Source: CAD feature listing. Evaluate the final solid. Frame: model axes, mm. A direction names the side the tool comes from. Give positions to 0.01 mm unless a question says otherwise; leave off trailing zeros. Order: outer loops, then holes, each group sorted by start corner. A loop starts at its lowest first (then second) coordinate and runs counter-clockwise, first axis right, second up.
Autodesk Inventor part; units mm, degrees
ref_plane "YZ Plane" through (0, 0, 0) normal (1, 0, 0) x (0, 1, 0)
ref_plane "XZ Plane" through (0, 0, 0) normal (0, 1, 0) x (-1, 0, 0)
ref_plane "XY Plane" through (0, 0, 0) normal (0, 0, 1) x (1, 0, 0)
sketch "Sketch1" plane through (0, 0, 0) normal (1, 0, 0) x (0, 1, 0)
  line L0 (444.5, 0) -> (444.5, -2.1042)
  line L1 (0, -2.1042) -> (0, 0)
  line L2 (0, -74.1174) -> (0, -66.8433)
  line L3 (0, 0) -> (82.55, 0)
  line L4 (82.55, 0) -> (82.55, -393.7)
  line L5 (82.55, -393.7) -> (0, -393.7)
  line L6 (0, -393.7) -> (0, 0)
  point P0 (25.4, -50.8)
  point P1 (25.4, -342.9)
  dimension "d2" = 82.55
  dimension "d3" = 393.7
  dimension "d4" = 50.8
  dimension "d5" = 25.4
  dimension "d6" = 50.8
  dimension "d7" = 25.4
extrude "Extrusion1" add sketch "Sketch1" along normal blind 6.35
sketch "Sketch3" plane through (6.35, 0, 0) normal (1, 0, 0) x (0, 0, -1)
  point P0 (0, 0)
sketch "Sketch4" plane through (6.35, 0, 0) normal (1, 0, 0) x (0, 0, -1)
  point P0 (0, 0)
chamfer "Chamfer1" distance 38.1 angle 45 1 edges at (3.175, 0, 0)
chamfer "Chamfer2" distance 38.1 angle 45 1 edges at (3.175, 0, -393.7)
sketch "Sketch5" plane through (0, 0, 0) normal (-1, 0, 0) x (0, 0, 1)
  line L0 (0, 82.55) -> (-393.7, 82.55)
  line L1 (-355.6, 0) -> (-393.7, 38.1)
  line L2 (-355.6, 0) -> (-38.1, 0)
  line L3 (0, 38.1) -> (-38.1, 0)
  line L4 (0, 38.1) -> (0, 82.55)
  line L5 (0, 82.55) -> (-393.7, 82.55)
  line L6 (-393.7, 82.55) -> (-393.7, 38.1)
  point P0 (0, 0)
  point P1 (-342.9, 38.1)
  point P2 (-50.8, 38.1)
  dimension "d16" = 50.8
  dimension "d17" = 38.1
  dimension "d18" = 38.1
  dimension "d19" = 50.8
hole "Hole1" at (0, 38.1, -342.9) at (0, 38.1, -50.8) direction (1, 0, 0) diameter 12.7254 end through all
sketch "Sketch7" plane through (0, 0, 0) normal (-1, 0, 0) x (0, 0, 1)
  line L0 (-38.1, 0) -> (-355.6, 0)
  line L1 (-393.7, 82.55) -> (-393.7, 38.1)
  line L2 (0, 38.1) -> (0, 82.55)
  line L3 (0, 82.55) -> (-393.7, 82.55)
  point P0 (0, 0)
  point P1 (-298.45, 10.0076)
  point P2 (-95.25, 10.0076)
  point P3 (-12.7, 78.8924)
  point P4 (-381, 78.8924)
  dimension "d42" = 10.0076
  dimension "d43" = 95.25
  dimension "d44" = 95.25
  dimension "d45" = 3.6576
  dimension "d46" = 12.7
  dimension "d47" = 12.7
  dimension "d82" = 3.6576
hole "Hole3" at (0, 78.8924, -381) at (0, 78.8924, -12.7) direction (1, 0, 0) diameter 4.7752 end through all
sketch "Sketch8" plane through (0, 0, 0) normal (-1, 0, 0) x (0, 0, 1)
  line L0 (0, 38.1) -> (0, 82.55)
  line L1 (0, 82.55) -> (-393.7, 82.55)
  line L2 (-355.6, 0) -> (-38.1, 0)
  line L3 (-393.7, 38.1) -> (-393.7, 82.55)
  point P0 (0, 0)
  point P1 (-171.45, 78.8924)
  point P2 (-222.25, 10.0076)
  dimension "d57" = 10.0076
  dimension "d128" = 222.25
hole "Hole4" at (0, 10.0076, -222.25) direction (1, 0, 0) diameter 3.556 end through all
sketch "Sketch10" plane through (0, 0, 0) normal (-1, 0, 0) x (0, 0, 1)
  circle A0 centre (-222.25, 44.45) radius 1.778
  circle A1 centre (-127, 44.45) radius 1.778
  line L0 (-393.7, 82.55) -> (0, 82.55)
  line L1 (-114.3619, 67.6125) -> (-112.4836, 67.6125)
  point P0 (0, 0)
  point P1 (-220.472, 44.45)
  point P2 (-128.778, 44.45)
  dimension "d108" = 38.1
  dimension "d109" = 38.1
hole "Hole6" at (0, 44.45, -127) at (0, 44.45, -220.472) at (0, 44.45, -128.778) at (0, 44.45, -222.25) direction (1, 0, 0) diameter 43.18 end through all
sketch "Sketch14" plane through (6.35, 0, 0) normal (1, 0, 0) x (0, 0, -1)
  arc A0 (127.889, 66.0217) -> (127.889, 22.8783) centre (127, 44.45) ccw
  arc A1 (127.889, 22.8783) -> (127.889, 66.0217) centre (128.778, 44.45) ccw
  arc A2 (221.361, 66.0217) -> (221.361, 22.8783) centre (220.472, 44.45) ccw
  arc A3 (221.361, 22.8783) -> (221.361, 66.0217) centre (222.25, 44.45) ccw
  line L0 (127.889, 66.0217) -> (127.889, 22.8783)
  line L1 (96.03, 44.45) -> (156.5626, 44.45)
  line L2 (221.361, 66.0217) -> (221.361, 22.8783)
  line L3 (190.5646, 36.322) -> (248.6345, 36.322)
  line L4 (127.889, 44.45) -> (103.886, 44.45)
  line L5 (103.886, 44.45) -> (103.886, 51.4604)
  line L6 (103.886, 51.4604) -> (103.886, 44.45)
  line L7 (103.886, 44.45) -> (103.886, 37.4396)
  line L8 (127.889, 44.45) -> (151.892, 44.45)
  line L9 (151.892, 44.45) -> (151.892, 37.4396)
  line L10 (151.892, 44.45) -> (151.892, 51.4604)
  line L11 (221.361, 51.4604) -> (197.358, 51.4604)
  line L12 (221.361, 51.4604) -> (245.364, 51.4604)
  line L13 (221.361, 37.4396) -> (197.358, 37.4396)
  line L14 (221.361, 37.4396) -> (245.364, 37.4396)
  circle A4 centre (103.886, 37.4396) radius 1.7526
  circle A5 centre (103.886, 51.4604) radius 1.7526
  circle A6 centre (151.892, 51.4604) radius 1.7526
  circle A7 centre (151.892, 37.4396) radius 1.7526
  circle A8 centre (197.358, 51.4604) radius 1.7526
  circle A9 centre (197.358, 37.4396) radius 1.7526
  circle A10 centre (245.364, 37.4396) radius 1.7526
  circle A11 centre (245.364, 51.4604) radius 1.7526
  point P0 (0, 0)
  dimension "d113" = 24.003
  dimension "d114" = 7.0104
  dimension "d115" = 7.0104
  dimension "d116" = 24.003
  dimension "d117" = 24.003
  dimension "d118" = 24.003
  dimension "d119" = 3.5052
  dimension "d120" = 3.5052
  dimension "d121" = 3.5052
  dimension "d122" = 3.5052
  dimension "d123" = 3.5052
extrude "Extrusion2" cut sketch "Sketch14" against normal blind 25.4 contours A9 L3 | A10 L3 | A9 L3 | L3 A10 | A4 | A5 | A6 | A7 | A8 | A11
thicken "Thicken1" operation add thickness 6.35 both sides no extend neighbours yes toward (0, 1, 0) faces at (2.1167, 82.55, -131.2333)
sketch "Sketch16" plane through (6.35, 0, 0) normal (1, 0, 0) x (0, 0, -1)
  line L0 (393.7, 88.9) -> (0, 88.9)
  line L1 (42.6019, 88.9) -> (52.7619, 88.9)
  line L2 (52.7619, 88.9) -> (52.7619, 78.74)
  line L3 (31.75, 78.74) -> (107.95, 78.74)
  line L4 (31.75, 78.74) -> (107.95, 78.74) construction
  point P0 (0, 0)
  dimension "d131" = 10.16
  dimension "d132" = 10.16
  dimension "d133" = 76.2
sketch "Sketch17" plane through (6.35, 0, 0) normal (1, 0, 0) x (0, 0, -1)
  circle A0 centre (139.7, 78.74) radius 1.778
  line L0 (393.7, 38.1) -> (393.7, 88.9)
  line L1 (393.7, 78.74) -> (304.8, 78.74)
  line L2 (393.7, 78.74) -> (482.6, 78.74) construction
  circle A1 centre (304.8, 78.74) radius 1.778
  point P0 (0, 0)
  dimension "d135" = 3.556
  dimension "d136" = 88.9
  dimension "d138" = 3.556
sketch "Sketch18" plane through (6.35, 0, 0) normal (1, 0, 0) x (0, 0, -1)
  line L0 (0, 0) -> (0, 10.0076)
  line L1 (0, 0) -> (10.0076, 0) construction
  line L2 (0, 10.0076) -> (101.6, 10.0076)
  line L3 (0, 10.0076) -> (101.6, 10.0076) construction
  line L4 (393.7, 10.0076) -> (292.1, 10.0076)
  line L5 (393.7, 10.0076) -> (495.3, 10.0076) construction
  circle A0 centre (101.6, 10.0076) radius 2.3876
  circle A1 centre (292.1, 10.0076) radius 2.3876
  dimension "d139" = 10.0076
  dimension "d141" = 101.6
  dimension "d143" = 101.6
  dimension "d145" = 4.7752
  dimension "d146" = 4.7752
hole "Hole10" at (6.35, 78.74, -107.95) direction (-1, 0, 0) diameter 3.556 depth 25.4 tip angle 118
hole "Hole11" at (6.35, 78.74, -304.8) direction (-1, 0, 0) diameter 3.556 depth 25.4 tip angle 118
hole "Hole12" at (6.35, 10.0076, -292.1) direction (-1, 0, 0) diameter 3.556 depth 25.4 tip angle 118
hole "Hole13" at (6.35, 10.0076, -101.6) direction (-1, 0, 0) diameter 3.556 depth 25.4 tip angle 118
sketch "Sketch19" plane through (6.35, 0, 0) normal (1, 0, 0) x (0, 0, -1)
  point P0 (0, 0)
sketch "Sketch20" plane through (6.35, 0, 0) normal (1, 0, 0) x (0, 0, -1)
  line L0 (0, 88.9) -> (0, 38.1)
  line L1 (38.1, 0) -> (0, 38.1)
  line L2 (38.1, 0) -> (355.6, 0)
  line L3 (393.7, 38.1) -> (355.6, 0)
  line L4 (393.7, 38.1) -> (393.7, 88.9)
  line L5 (393.7, 88.9) -> (0, 88.9)
  line L6 (0, 63.5) -> (19.05, 63.5)
  line L7 (19.05, 88.9) -> (19.05, 69.85)
  line L8 (56.4869, 0) -> (56.4869, 19.05)
  circle A0 centre (50.8, 38.1) radius 6.3627
  circle A1 centre (50.8, 38.1) radius 6.3627
  line L9 (44.4412, 37.8775) -> (33.0112, 37.8775)
  line L10 (50.5074, 44.456) -> (50.5074, 55.886)
  line L11 (57.1622, 38.1805) -> (68.5922, 38.1805)
  circle A2 centre (103.886, 37.4396) radius 1.7526
  line L12 (102.1334, 37.4396) -> (90.7034, 37.4396)
  line L13 (80.4606, 88.9) -> (80.4606, 69.85)
  line L14 (68.5922, 69.85) -> (90.7034, 69.85)
  line L15 (90.7034, 69.85) -> (90.7034, 19.05)
  line L16 (90.7034, 19.05) -> (68.5922, 19.05)
  line L17 (68.5922, 19.05) -> (68.5922, 69.85)
  line L18 (19.05, 69.85) -> (33.0112, 69.85)
  line L19 (33.0112, 69.85) -> (33.0112, 33.0112)
  line L20 (33.0112, 33.0112) -> (19.05, 33.0112)
  line L21 (19.05, 33.0112) -> (19.05, 69.85)
  line L22 (19.05, 33.0112) -> (33.0112, 33.0112)
  line L23 (33.0112, 33.0112) -> (33.0112, 19.05)
  line L24 (33.0112, 19.05) -> (19.05, 33.0112)
  line L25 (33.0112, 19.05) -> (33.0112, 33.0112)
  line L26 (19.05, 33.0112) -> (33.0112, 33.0112)
  line L27 (19.05, 33.0112) -> (33.0112, 19.05)
  line L28 (33.0112, 33.0112) -> (33.0112, 69.85)
  line L29 (33.0112, 69.85) -> (19.05, 69.85)
  line L30 (19.05, 69.85) -> (19.05, 33.0112)
  point P0 (0, 0)
  dimension "d183" = 19.05
  dimension "d184" = 19.05
  dimension "d185" = 19.05
  dimension "d186" = 11.43
  dimension "d187" = 11.43
  dimension "d188" = 11.43
  dimension "d189" = 11.43
  dimension "d190" = 19.05
extrude "Extrusion3" cut sketch "Sketch20" against normal blind 25.4 contours L14 L15 L16 L17
extrude "Extrusion4" cut sketch "Sketch20" against normal blind 25.4 contours L21 L18 L19 L20 | L20 L23 L24
sketch "Sketch21" plane through (6.35, 0, 0) normal (1, 0, 0) x (0, 0, -1)
  circle A0 centre (151.892, 51.4604) radius 1.7526
  line L0 (38.1, 0) -> (355.6, 0)
  circle A1 centre (197.358, 51.4604) radius 1.7526
  line L1 (393.7, 88.9) -> (0, 88.9)
  line L2 (0, 88.9) -> (393.7, 88.9)
  line L3 (175.7731, 88.9) -> (175.7731, 69.85)
  line L4 (153.6446, 51.4604) -> (165.0746, 51.4604)
  circle A2 centre (197.358, 51.4604) radius 1.7526
  line L5 (195.6055, 51.4771) -> (184.1755, 51.4771)
  line L6 (355.6, 0) -> (38.1, 0)
  line L7 (175.7731, 0) -> (175.7731, 19.05)
  line L8 (165.0746, 69.85) -> (184.1755, 69.85)
  line L9 (184.1755, 69.85) -> (184.1755, 19.05)
  line L10 (184.1755, 19.05) -> (165.0746, 19.05)
  line L11 (165.0746, 19.05) -> (165.0746, 69.85)
  circle A3 centre (245.364, 51.4604) radius 1.7526
  circle A4 centre (245.364, 37.4396) radius 1.7526
  circle A5 centre (342.9, 38.1) radius 6.3627
  line L12 (267.1323, 0) -> (267.1323, 19.05)
  line L13 (267.1323, 88.9) -> (267.1323, 69.85)
  line L14 (247.1166, 51.4604) -> (258.5466, 51.4604)
  line L15 (336.5373, 38.1) -> (325.1073, 38.1)
  line L16 (258.5466, 69.85) -> (325.1073, 69.85)
  line L17 (325.1073, 69.85) -> (325.1073, 19.05)
  line L18 (325.1073, 19.05) -> (258.5466, 19.05)
  line L19 (258.5466, 19.05) -> (258.5466, 69.85)
  point P0 (0, 0)
  dimension "d195" = 19.05
  dimension "d196" = 11.43
  dimension "d197" = 11.43
  dimension "d198" = 19.05
  dimension "d199" = 19.05
  dimension "d200" = 19.05
  dimension "d201" = 11.43
  dimension "d202" = 11.43
extrude "Extrusion5" cut sketch "Sketch21" against normal blind 25.4 contours L10 L11 L8 L9
extrude "Extrusion6" cut sketch "Sketch21" against normal blind 25.4 contours L18 L19 L16 L17
sketch "Sketch22" plane through (6.35, 0, 0) normal (1, 0, 0) x (0, 0, -1)
  line L0 (393.7, 38.1) -> (393.7, 88.9)
  line L1 (361.8045, 88.9) -> (361.8045, 69.85)
  circle A0 centre (342.9, 38.1) radius 6.3627
  line L2 (349.2627, 38.1) -> (360.6927, 38.1)
  line L3 (393.7, 39.2414) -> (374.65, 39.2414)
  line L4 (360.6927, 69.85) -> (374.65, 69.85)
  line L5 (374.65, 69.85) -> (374.65, 27.244)
  line L6 (374.65, 27.244) -> (360.6927, 27.244)
  line L7 (360.6927, 27.244) -> (360.6927, 69.85)
  line L8 (360.6927, 27.244) -> (360.6927, 13.2867)
  line L9 (360.6927, 13.2867) -> (374.65, 27.244)
  line L10 (355.6, 0) -> (393.7, 38.1)
  point P0 (0, 0)
  dimension "d207" = 19.05
  dimension "d208" = 11.43
  dimension "d209" = 19.05
extrude "Extrusion7" cut sketch "Sketch22" against normal blind 25.4 contours L4 L5 L6 L7 | L6 L9 L8
properties part number "DriveTrainPlate"
1) Ray query, L1, parallel to Z at x = 5.25, y = 68; L2, parallel to Z at x = 1.75, y = 9.5; L3, parallel to Y at x = 1.25, z = -79. Return the intervals inside material, ascending.
Checks:
L1: z = -393.7 to -374.65, -360.69 to -325.11, -258.55 to -184.18, -165.07 to -90.7, -68.59 to -33.01, -19.05 to 0
L2: z = -365.1 to -293.8, -290.4 to -223.95, -220.55 to -103.3, -99.9 to -28.6
L3: y = 0 to 19.05, 69.85 to 88.9
2) Section query A-A on z = -50.8. Output: boundary loops of the cut face in (x, y).
Checks:
outline: (0, 0) - (6.35, 0) - (6.35, 31.74) - (0, 31.74) - close; (0, 44.46) - (6.35, 44.46) - (6.35, 88.9) - (0, 88.9) - close
3) Section query B-B on z = -118. Output: boundary loops of the cut face in (x, y), and give its area (3 significant figures).
Checks:
outline: (0, 0) - (6.35, 0) - (6.35, 24.83) - (0, 24.83) - close; (0, 64.07) - (6.35, 64.07) - (6.35, 88.9) - (0, 88.9) - close
area: 315 mm2
4) Reachability of faces 4 (the face through (3, 69.85, -291)), 5 (the face through (0, 44, -194)) from +Z, -Z, +X, -X, +Y, -Y: full face, straight path, thin tool, end or side. Return the list, or none.
Checks:
face 4: +X, -X
face 5: +Z, -Z, -X, +Y, -Y
5) Pull-direction query (Z, two-part tool) for faces 1 (the face through (3.1, 18.8, -374.4)), 2 (the face through (3, 44, -258.547)), 3 (the face through (3, 0, -199)); classes: +Z half, -Z half, draft (parallel to the pull), parting line (faces both ways), or undercut.
Checks:
face 1: -Z half
face 2: undercut
face 3: draft
6) Section query C-C on x = 1.25. State how many separate pieces and enclosed holes the cut face has, and give its area (3 significant figures).
Checks:
separate pieces: 1
enclosed holes: 24
area: 23,300 mm2
7) First-contact query: pin 1 Ø3 at (y, z) = (51.46, -151.89) entering from +X; pin 2 Ø1.5 at (x, y) = (2, 28) entering from +Z. Flat tips, straight axial feed; report the tip coordinate or a pass-through.
Checks:
pin 1: passes through
pin 2: stops at z = -9.35
